Autodesk Inventor part; units mm, degrees
ref_plane "YZ Plane" through (0, 0, 0) normal (1, 0, 0) x (0, 1, 0)
ref_plane "XZ Plane" through (0, 0, 0) normal (0, 1, 0) x (-1, 0, 0)
ref_plane "XY Plane" through (0, 0, 0) normal (0, 0, 1) x (1, 0, 0)
sketch "Sketch1" plane through (0, 0, 0) normal (0, 0, 1) x (1, 0, 0)
  arc A0 (-10.5987, 11.9888) -> (10.5987, 11.9888) centre (0, 0) ccw
  line L0 (-10.5987, 11.9888) -> (10.5987, 11.9888)
  arc A1 (12.5617, -3.3659) -> (12.5617, 3.3659) centre (0, 0) ccw construction
  arc A2 (13.5185, -3.6223) -> (13.5185, 3.6223) centre (0, 0) ccw
  arc A3 (11.6048, -3.1095) -> (11.6048, 3.1095) centre (0, 0) ccw
  arc A4 (11.6048, -3.1095) -> (13.5185, -3.6223) centre (12.5617, -3.3659) ccw
  arc A5 (13.5185, 3.6223) -> (11.6048, 3.1095) centre (12.5617, 3.3659) ccw
  line L1 (0, 0) -> (20.2969, 0) construction
  arc A6 (3.6223, -13.5185) -> (9.8962, -9.8962) centre (0, 0) ccw
  arc A7 (3.1095, -11.6048) -> (3.6223, -13.5185) centre (3.3659, -12.5617) ccw
  arc A8 (3.1095, -11.6048) -> (8.4953, -8.4953) centre (0, 0) ccw
  arc A9 (9.8962, -9.8962) -> (8.4953, -8.4953) centre (9.1958, -9.1958) ccw
  arc A10 (3.3659, -12.5617) -> (9.1958, -9.1958) centre (0, 0) ccw construction
  arc A11 (-9.8962, -9.8962) -> (-3.6223, -13.5185) centre (0, 0) ccw
  arc A12 (-8.4953, -8.4953) -> (-9.8962, -9.8962) centre (-9.1958, -9.1958) ccw
  arc A13 (-8.4953, -8.4953) -> (-3.1095, -11.6048) centre (0, 0) ccw
  arc A14 (-3.6223, -13.5185) -> (-3.1095, -11.6048) centre (-3.3659, -12.5617) ccw
  arc A15 (-9.1958, -9.1958) -> (-3.3659, -12.5617) centre (0, 0) ccw construction
  arc A16 (-13.5185, 3.6223) -> (-13.5185, -3.6223) centre (0, 0) ccw
  arc A17 (-11.6048, 3.1095) -> (-13.5185, 3.6223) centre (-12.5617, 3.3659) ccw
  arc A18 (-11.6048, 3.1095) -> (-11.6048, -3.1095) centre (0, 0) ccw
  arc A19 (-13.5185, -3.6223) -> (-11.6048, -3.1095) centre (-12.5617, -3.3659) ccw
  arc A20 (-12.5617, 3.3659) -> (-12.5617, -3.3659) centre (0, 0) ccw construction
  dimension "d0" = 27.9908
  dimension "d1" = 16.002
  dimension "d2" = 30
  dimension "d3" = 13.0048
  dimension "d4" = 0.9906
  dimension "d7" = 180
extrude "Extrusion1" add sketch "Sketch1" along normal blind 5.9944
sketch "Sketch2" plane through (0, 0, 0) normal (0, 0, -1) x (-1, 0, 0)
  circle A0 centre (0, 0) radius 5.9944
  dimension "d11" = 11.9888
extrude "Extrusion2" add sketch "Sketch2" along normal blind 1.9812
hole "Hole1" at (0, 0, 5.9944) direction (0, 0, -1) diameter 8.001 end through all counterbore diameter 9.9822 counterbore depth 1.9812
sketch "Sketch3" plane through (0, 0, 5.9944) normal (0, 0, 1) x (1, 0, 0)
  point P0 (0, 0)
  point P1 (8.9916, 0)
  dimension "d23" = 8.9916
hole "Hole2" at (8.9916, 0, 5.9944) direction (0, 0, -1) diameter 1.4224 depth 5.6896 tip angle 118 counterbore diameter 2.9972 counterbore depth 0.9906
pattern_circular "Circular Pattern1" count 6 over 360 about axis through (0, 0, 0) along (0, 0, 1) of "Hole2"
chamfer "Chamfer1" distance 0.9906 angle 30 1 edges at (0, 4.9911, 5.9944) measured on face at (0.4016, -4.9749, 5.334)
properties part number "Ch5_tut1"
Geometry: final body of the model. Coordinates: model frame, mm. A direction names the side the tool comes from. Give positions to 0.01 mm unless a question says otherwise; leave off trailing zeros. Write each loop counter-clockwise with the first axis right and the second up, starting at its lowest first coordinate (ties: lowest second). Pieces come first, ordered by that corner, then holes. Notation, with made-up numbers: M -0.5,9.25 L 13.5,9.25 A32 ccw 13.5,36.25 Z; hole C 22.5,-26.75 d2. An arc over 180 degrees is marked long. Answer in a Markdown table with one row per item. Add a question column.
(1) Section B-B on z = 5.5. State how many separate pieces and enclosed holes the cut face has, and give its area (3 significant figures).
(2) Section C-C on y = -12.5. Return loops of the section in (x, z), and give its area (3 significant figures).
(3) Mould query, pull axis Y, two halves, no side actions, for faces 1 (the cylindrical face through (5.095, 8.169, 2.621)), 2 (the cylindrical face through (-5.718, -1.801, -0.977)). Classes: +Y half, -Y half, draft (parallel to the pull), parting line (faces both ways), or undercut.
(4) Section A-A on x = 0. Return loops of the section in (y, z).
(5) First-contact query: pin 1 (4 mm diameter, centred on x = 11.5, y = 7, fed in from -Z); pin 2 (3 mm diameter, centred on y = -11, z = 0.5, fed in from +X); pin 3 (1 mm diameter, centred on y = -6, z = 0.5, fed in from -X). Flat tips, straight axial feed; report the tip coordinate or a pass-through.
(6) Ray query, line 1 (Y direction, x = -5, z = 1); line 2 (Y direction, x = 9, z = 1); line 3 (X direction, y = 2.5, z = 2.5). Return the intervals inside material, ascending.
(7) Reachability of faces 3 (the cylindrical face through (6.05, -10.38, 2.96)), 4 (the cylindrical face through (-5.5, 8.9, 5.5)) from +Z, -Z, +X, -X, +Y, -Y: full face, straight path, thin tool, end or side. Return the list, or none.
Result set:
| question | item | result |
|---|---|---|
| 1 | separate pieces | 1 |
| 1 | enclosed holes | 11 |
| 1 | area | 550 mm^2 |
| 2 | outline | M -9.99,0 L -6.29,0 L -6.29,5.99 L -9.99,5.99 Z; M -2.38,0 L 2.38,0 L 2.38,5.99 L -2.38,5.99 Z; M 6.29,0 L 9.99,0 L 9.99,5.99 L 6.29,5.99 Z |
| 2 | area | 72.8 mm^2 |
| 3 | face 1 | undercut |
| 3 | face 2 | parting line |
| 4 | outline | M -16,0 L -5.99,0 L -5.99,-1.98 L -4,-1.98 L -4,4.01 L -4.99,4.01 L -4.99,5 L -5.56,5.99 L -16,5.99 Z; M 4,-1.98 L 5.99,-1.98 L 5.99,0 L 11.99,0 L 11.99,5.99 L 5.56,5.99 L 4.99,5 L 4.99,4.01 L 4,4.01 Z |
| 5 | pin 1 | stops at z = 0 |
| 5 | pin 2 | stops at x = 12.88 |
| 5 | pin 3 | stops at x = -15.03 |
| 6 | line 1 | y = -15.2 to -13.07, -10.92 to -8.29, -7.29 to 7.29, 8.29 to 11.99 |
| 6 | line 2 | y = -13.23 to -10.72, -8.22 to -0.71, 0.71 to 11.99 |
| 6 | line 3 | x = -15.81 to -13.77, -11.75 to -3.12, 3.12 to 11.75, 13.77 to 15.81 |
| 7 | face 3 | +Z, -Z |
| 7 | face 4 | +Z |
